Verification items for the finished model (mm, model axes). A direction names the side the tool comes from. Give positions to 0.01 mm unless a question says otherwise; leave off trailing zeros. Order: outer loops, then holes, each group sorted by start corner. A loop starts at its lowest first (then second) coordinate and runs counter-clockwise, first axis right, second up.
from build123d import *

# Parameters (mm, degrees)
BOSS_EXTRUDE1_DEPTH = 700
CUT_EXTRUDE1_REACH  = 705.562
SKETCH2_R           = 6


with BuildPart() as part:
    # Sketch1 → Boss-Extrude1 (new, symmetric)
    with BuildSketch(Plane(origin=(0, 0, 0), x_dir=(1, 0, 0), z_dir=(0, 1, 0))):
        with BuildLine():
            Line((0, 0), (-50, 0))
            Line((-50, 0), (-50, -2.5))
            ThreePointArc((-50, -2.5), (-48.974873734, -4.974873734), (-46.5, -6))
            Line((-46.5, -6), (-13, -6))
            ThreePointArc((-13, -6), (-8.050252532, -8.050252532), (-6, -13))
            Line((-6, -13), (-6, -46.5))
            ThreePointArc((-6, -46.5), (-4.974873734, -48.974873734), (-2.5, -50))
            Line((-2.5, -50), (0, -50))
            Line((0, -50), (0, 0))
        make_face()
    extrude(amount=BOSS_EXTRUDE1_DEPTH, both=True)

    # Sketch2 → Cut-Extrude1 (cut, up to next)
    with BuildSketch(Plane(origin=(0, 0, 0), x_dir=(-1, 0, 0), z_dir=(0, 0, -1)), mode=Mode.PRIVATE) as cut_extrude1_sk1:
        with Locations((30, 52.92)):
            Circle(SKETCH2_R)
    cut_extrude1_tool1 = extrude(cut_extrude1_sk1.sketch, amount=-CUT_EXTRUDE1_REACH, mode=Mode.PRIVATE) & part.part
    # Sketch2 → Cut-Extrude1 (cut, up to next)
    with BuildSketch(Plane(origin=(0, 0, 0), x_dir=(-1, 0, 0), z_dir=(0, 0, -1)), mode=Mode.PRIVATE) as cut_extrude1_sk2:
        with Locations((30, -52.92)):
            Circle(SKETCH2_R)
    cut_extrude1_tool2 = extrude(cut_extrude1_sk2.sketch, amount=-CUT_EXTRUDE1_REACH, mode=Mode.PRIVATE) & part.part
    add(cut_extrude1_tool1.solids().sort_by_distance((-30, 52.92, 0))[0], mode=Mode.SUBTRACT)
    add(cut_extrude1_tool2.solids().sort_by_distance((-30, -52.92, 0))[0], mode=Mode.SUBTRACT)


solid = part.part
(1) Section check A-A, the plane y = 584.5. Enter the section's corners in (x, z).
Solved:
outline: (-50, 0) - (0, 0) - (0, 50) - (-2.5, 50) arc R3.5 ccw to (-6, 46.5) - (-6, 13) arc R7 cw to (-13, 6) - (-46.5, 6) arc R3.5 ccw to (-50, 2.5) - close
(2) Scan lines: line 1 (Y direction, x = -30, z = 3); line 2 (X direction, y = 19, z = 30); line 3 (Z direction, x = -41, y = 550). Record each from-to range of solid material in increasing order.
Solved:
line 1: y = -700 to -58.92, -46.92 to 46.92, 58.92 to 700
line 2: x = -6 to 0
line 3: z = 0 to 6
(3) Set-up check for faces 1 (the flat face through (-25, 10, 0)), 2 (the flat face through (-6, 10, 30)): record each of +Z, -Z, +X, -X, +Y, -Y from which the full face is reachable in a straight line by a thin tool's end or side.
Solved:
face 1: -Z, +X, -X, +Y, -Y
face 2: +Z, -X, +Y, -Y
(4) Section check B-B, the plane z = 38.5. Enter the section's corners in (x, y), then the cut area to 3 significant figures.
Solved:
outline: (-6, -700) - (0, -700) - (0, 700) - (-6, 700) - close
area: 8,400 mm2
(5) Go/stop test with flat-tipped pins: pin 1 (19 mm diameter, centred on x = -30, y = 52.92, fed in from +Z); pin 2 (8 mm diameter, centred on y = 46, z = 35, fed in from -X); pin 3 (12 mm diameter, centred on x = -25, y = 179.5, fed in from -Z); pin 4 (10 mm diameter, centred on x = -12, y = 191, fed in from +Z). Record where each tip stops, or that it passes through.
Solved:
pin 1: stops at z = 6
pin 2: stops at x = -6
pin 3: stops at z = 0
pin 4: stops at z = 9.39
